The model under review builds one solid part; all positions refer to its coordinate system, in mm. Round coordinates to 2 decimals unless told otherwise and drop trailing zeros. Loops run counter-clockwise (first coordinate to the right, second up) from the corner with the lowest first, then second, coordinate; pieces in that order, holes last. Notation, with made-up numbers: (-39, -9.75) - (-11, -9.75) arc R10 ccw to (-11, -1.75) - close; hole circle Ø6 at (-17.5, -13.75). An arc over 180 degrees is marked (long way). Answer as CSV lines item,"result".
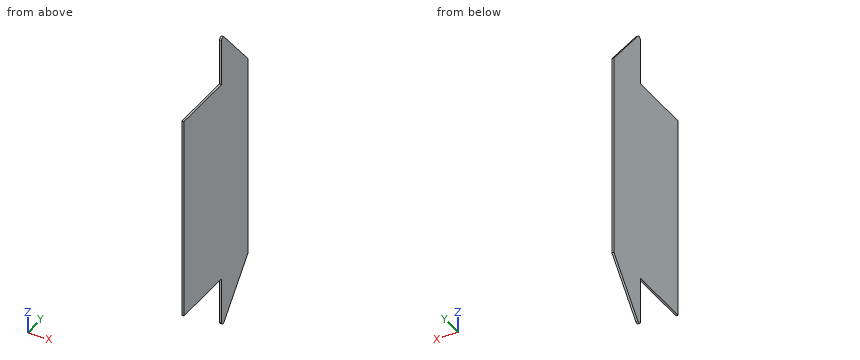
from build123d import *

# Parameters (mm, degrees)
BOSS_EXTRUDE1_DEPTH = 6.35
FILLET1_R           = 7.62


with BuildPart() as part:
    # Sketch1 → Boss-Extrude1 (new body)
    with BuildSketch(Plane(origin=(0, 0, 0), x_dir=(0, 0, -1), z_dir=(1, 0, 0))):
        Polygon((330, 101.6), (482.4, 101.6), (499.846481614, 101.6), (486.481701322, 112.814382214), (330, 244.118120079), (-330, 244.118120079), (-499.846481614, 101.6), (-482.4, 101.6), (-330, 101.6), (-330, -101.6), (330, -101.6), align=None)
    extrude(amount=BOSS_EXTRUDE1_DEPTH)

    # Fillet1
    fillet1_edges = [part.edges().sort_by_distance(p)[0] for p in [
        (3.175, 101.6, 499.846481614),
        (3.175, 101.6, -499.846481614),
    ]]
    fillet(fillet1_edges, radius=FILLET1_R)


solid = part.part
1. Take a section at B-B (z = -395.5). State the section outline as (x, y) points.
Numbers:
outline,"(0, 101.6) - (6.35, 101.6) - (6.35, 189.16) - (0, 189.16) - close"
2. Take a section at A-A (y = 68.5). State the section outline as (x, z) points, plus the area to 3 significant figures.
Numbers:
outline,"(0, -330) - (6.35, -330) - (6.35, 330) - (0, 330) - close"
area,"4,190 mm²"
3. Clearance check with flat-ended pins moving along their axes: pin 1 (1 mm diameter, centred on x = 4, y = 167, fed in from -Z); pin 2 (2 mm diameter, centred on y = 49, z = -214.5, fed in from -X). State where each tip first meets the part, or that it passes through.
Numbers:
pin 1,"stops at z = -422.5"
pin 2,"stops at x = 0"
4. Wall thickness on probe 1 along Z at (x, y) = (5.5, 35); probe 2 along Z at (x, y) = (6, 165.5); probe 3 along Y at (x, z) = (0.75, 384.5): over which ranges is each line inside the solid? List them lowest first.
Numbers:
probe 1,"z = -330 to 330"
probe 2,"z = -423.69 to 423.69"
probe 3,"y = 101.6 to 198.39"
